Build history of the part. All positions in model axes, mm. Face numbers are marked on the shaded views. A direction names the side the tool comes from. Round coordinates to 2 decimals unless told otherwise and drop trailing zeros. Write each loop counter-clockwise with the first axis right and the second up, starting at its lowest first coordinate (ties: lowest second). Pieces come first, ordered by that corner, then holes.
1) Wall check: probe 1 along Z at (x, y) = (19.5, -4.5); probe 2 along Y at (x, z) = (5, 4.7); probe 3 along Y at (x, z) = (15.5, -4). Give the ranges that are in metal, low to high.
2) Saw through at C-C (x = 5). Write the cut outline in (y, z).
3) Which spindle directions (+Z, -Z, +X, -X, +Y, -Y) get a long thin tool onto all of the face, cutting with end or side? Do the marked faces 1, 2, 3 and 4. Say none if no direction does.
4) Saw through at B-B (y = -11.5). Write the cut outline in (x, z).
5) Flat gauge pins, fed straight in: pin 1 (2 mm diameter, centred on x = 15.5, y = -12, fed in from -Z); pin 2 (4 mm diameter, centred on x = 5.5, y = 1, fed in from -Z); pin 3 (3 mm diameter, centred on y = -3.5, z = -9.5, fed in from -X); pin 4 (2 mm diameter, centred on y = -10.5, z = 10.5, fed in from -X). Where does each tip first touch, or does it go through?
6) Saw through at A-A (z = 6). Write the cut outline in (x, y), plus the area to 3 significant figures.
7) Saw through at D-D (y = 0). Write the cut outline in (x, z).
8) Pull direction Y, two halves, no side cores. Call the marked faces 5, 6 and 7: +Y half, -Y half, draft (parallel to the pull), parting line (faces both ways), or undercut.
from build123d import *

# Parameters (mm, degrees)
BOSS_EXTRUDE1_DEPTH = 12
CUT_EXTRUDE1_REACH  = 33.988
SKETCH4_R           = 1.65
SKETCH4_3_W         = 10
SKETCH4_3_H         = 5
SKETCH4_3_R         = 1.65
CUT_EXTRUDE3_DEPTH  = 7
CUT_EXTRUDE2_REACH  = 26.698
SKETCH5_R           = 3.75
SKETCH6_W           = 4
SKETCH6_H           = 14
BOSS_EXTRUDE2_DEPTH = 24
SKETCH7_W           = 20
SKETCH7_H           = 14
CUT_EXTRUDE4_DEPTH  = 10


with BuildPart() as part:
    # Sketch3 → Boss-Extrude1 (new, symmetric)
    with BuildSketch(Plane.XY):
        Polygon((-21, 2.5), (-12.339745962, -2.5), (21, -2.5), (21, 2.5), align=None)
    extrude(amount=BOSS_EXTRUDE1_DEPTH, both=True)

    # Sketch4 → Cut-Extrude1 (cut, up to next)
    with BuildSketch(Plane.XY.offset(12), mode=Mode.PRIVATE) as cut_extrude1_sk1:
        with Locations((5, 0)):
            Circle(SKETCH4_R)
    cut_extrude1_tool1 = extrude(cut_extrude1_sk1.sketch, amount=-CUT_EXTRUDE1_REACH, mode=Mode.PRIVATE) & part.part
    add(cut_extrude1_tool1.solids().sort_by_distance((5, 0, 12))[0], mode=Mode.SUBTRACT)

    # Sketch4<3> → Cut-Extrude3 (cut)
    with BuildSketch(Plane.XY.offset(12)):
        with Locations((5, 0)):
            Rectangle(SKETCH4_3_W, SKETCH4_3_H)
        with Locations((5, 0)):
            Circle(SKETCH4_3_R, mode=Mode.SUBTRACT)
    cut_extrude3 = extrude(amount=-CUT_EXTRUDE3_DEPTH, mode=Mode.SUBTRACT)

    # Mirror1: Cut-Extrude3 across plane
    add(cut_extrude3.mirror(Plane.XY), mode=Mode.SUBTRACT)

    # Sketch5 → Cut-Extrude2 (cut, up to next)
    with BuildSketch(Plane(origin=(0, 2.5, 0), x_dir=(1, 0, 0), z_dir=(0, 1, 0)), mode=Mode.PRIVATE) as cut_extrude2_sk1:
        with Locations(Location((5, 0, 0), (0, 0, 270))):
            Circle(SKETCH5_R)
    cut_extrude2_tool1 = extrude(cut_extrude2_sk1.sketch, amount=-CUT_EXTRUDE2_REACH, mode=Mode.PRIVATE) & part.part
    add(cut_extrude2_tool1.solids().sort_by_distance((5, 2.5, 0))[0], mode=Mode.SUBTRACT)

    # Sketch6 → Boss-Extrude2 (add)
    with BuildSketch(Plane.XY.offset(12)):
        with Locations((19, -9.5)):
            Rectangle(SKETCH6_W, SKETCH6_H)
    extrude(amount=-BOSS_EXTRUDE2_DEPTH)

    # Sketch7 → Cut-Extrude4 (cut)
    with BuildSketch(Plane(origin=(21, 0, 0), x_dir=(0, 0, -1), z_dir=(1, 0, 0))):
        with Locations((0, -9.5)):
            Rectangle(SKETCH7_W, SKETCH7_H)
    extrude(amount=-CUT_EXTRUDE4_DEPTH, mode=Mode.SUBTRACT)


solid = part.part
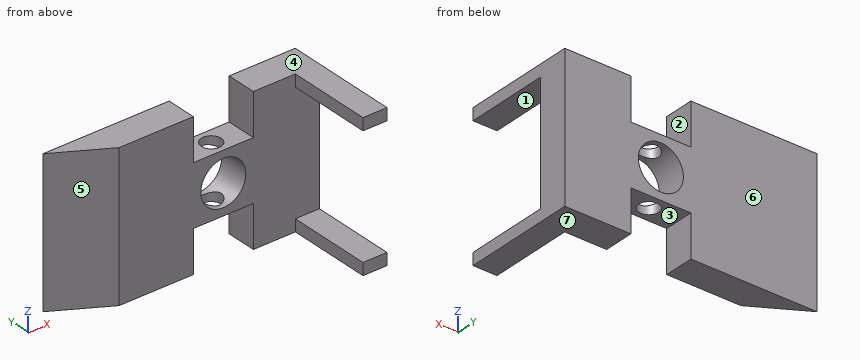
Evaluation:
1. probe 1: z = -12 to -10, 10 to 12
1. probe 2: y = -2.5 to -1.65, 1.65 to 2.5
1. probe 3: y = -2.5 to 2.5
2. outline: (-2.5, -5) - (-1.65, -5) - (-1.65, -3.75) - (-2.5, -3.75) - close; (-2.5, 3.75) - (-1.65, 3.75) - (-1.65, 5) - (-2.5, 5) - close; (1.65, -5) - (2.5, -5) - (2.5, -3.75) - (1.65, -3.75) - close; (1.65, 3.75) - (2.5, 3.75) - (2.5, 5) - (1.65, 5) - close
3. face 1: +X, -X, -Y
3. face 2: +Z, +Y, -Y
3. face 3: -Z, +Y, -Y
3. face 4: +Z, +X, -X, +Y, -Y
4. outline: (17, -12) - (21, -12) - (21, -10) - (17, -10) - close; (17, 10) - (21, 10) - (21, 12) - (17, 12) - close
5. pin 1: passes through
5. pin 2: stops at z = -5
5. pin 3: stops at x = -13.21
5. pin 4: stops at x = 17
6. outline: (-21, 2.5) - (-12.34, -2.5) - (0, -2.5) - (0, 2.5) - close; (10, -2.5) - (21, -2.5) - (21, 2.5) - (10, 2.5) - close
6. area: 138 mm2
7. outline: (-16.67, -12) - (0, -12) - (0, -5) - (3.35, -5) - (3.35, -3.37) arc R3.75 cw to (3.35, 3.37) - (3.35, 5) - (0, 5) - (0, 12) - (-16.67, 12) - close; (6.65, -5) - (10, -5) - (10, -12) - (21, -12) - (21, 12) - (10, 12) - (10, 5) - (6.65, 5) - (6.65, 3.37) arc R3.75 cw to (6.65, -3.37) - close
8. face 5: -Y half
8. face 6: +Y half
8. face 7: draft
